from build123d import *

# Parameters (mm, degrees)
SKETCH_1_W          = 12.5
SKETCH_1_H          = 12.5
EXTRUDE_412_DEPTH   = 4.5
FILLET_1_R          = 1.5
FILLET_2_R          = 1
SKETCH_2_W          = 15
SKETCH_2_H          = 15
EXTRUDE_1329_DEPTH  = 0.5
FILLET_3_R          = 3
CUT_EXTRUDE_1_DEPTH = 0.4
FILLET_4_R          = 0.5


with BuildPart() as part:
    # Эскиз1 → Extrude 412 (new body)
    with BuildSketch(Plane.XY):
        Rectangle(SKETCH_1_W, SKETCH_1_H)
    extrude(amount=EXTRUDE_412_DEPTH)

    # Скругление1
    fillet_1_edges = [part.edges().sort_by_distance(p)[0] for p in [
        (-6.25, 6.25, 2.25),
        (6.25, 6.25, 2.25),
        (6.25, -6.25, 2.25),
        (-6.25, -6.25, 2.25),
    ]]
    fillet(fillet_1_edges, radius=FILLET_1_R)

    # Скругление2
    fillet_2_edges = [part.edges().sort_by_distance(p)[0] for p in [
        (6.25, 0, 4.5),
        (0, -6.25, 4.5),
        (-6.25, 0, 4.5),
        (0, 6.25, 4.5),
        (-5.810660172, -5.810660172, 4.5),
        (-5.810660172, 5.810660172, 4.5),
        (5.810660172, 5.810660172, 4.5),
        (5.810660172, -5.810660172, 4.5),
    ]]
    fillet(fillet_2_edges, radius=FILLET_2_R)

    # Эскиз2 → Extrude 1329 (add)
    with BuildSketch(Plane(origin=(0, 0, 0), x_dir=(-1, 0, 0), z_dir=(0, 0, -1))):
        Rectangle(SKETCH_2_W, SKETCH_2_H)
    extrude(amount=-EXTRUDE_1329_DEPTH)

    # Скругление3
    fillet_3_edges = [part.edges().sort_by_distance(p)[0] for p in [
        (7.5, -7.5, 0.25),
        (7.5, 7.5, 0.25),
        (-7.5, 7.5, 0.25),
        (-7.5, -7.5, 0.25),
    ]]
    fillet(fillet_3_edges, radius=FILLET_3_R)

    # Эскиз4 → Вырез-Вытянуть1 (cut)
    with BuildSketch(Plane.XY.offset(4.5)):
        Polygon((-3.61015121, 1.724032908), (-3.61015121, -1.724032908), (-1.580654119, -1.724032908), (0.195408328, -3.515449311), (0.195408328, 3.515449311), (-1.580654119, 1.724032908), align=None)
        with BuildLine():
            ThreePointArc((1.529185986, -1.383686517), (1.749358373, 0), (1.529185986, 1.383686517))
            ThreePointArc((1.529185986, 1.383686517), (1.758587632, 1.835514539), (2.210415654, 1.606112893))
            ThreePointArc((2.210415654, 1.606112893), (2.465980556, 0), (2.210415654, -1.606112893))
            ThreePointArc((2.210415654, -1.606112893), (1.758587632, -1.835514539), (1.529185986, -1.383686517))
        make_face()
        with BuildLine():
            ThreePointArc((2.847646844, -3.007485014), (3.609370922, 0), (2.847646844, 3.007485014))
            ThreePointArc((2.847646844, 3.007485014), (3.055453428, 3.70569516), (3.753663574, 3.497888576))
            ThreePointArc((3.753663574, 3.497888576), (4.639595154, 0), (3.753663574, -3.497888576))
            ThreePointArc((3.753663574, -3.497888576), (3.055453428, -3.70569516), (2.847646844, -3.007485014))
        make_face()
    extrude(amount=-CUT_EXTRUDE_1_DEPTH, mode=Mode.SUBTRACT)

    # Скругление4
    fillet_4_edges = [part.edges().sort_by_distance(p)[0] for p in [
        (0.195408328, 3.515449311, 4.3),
        (0.195408328, -3.515449311, 4.3),
    ]]
    fillet(fillet_4_edges, radius=FILLET_4_R)


solid = part.part
Verification items for the finished model (mm, model axes). A direction names the side the tool comes from. Give positions to 0.01 mm unless a question says otherwise; leave off trailing zeros. Write each loop counter-clockwise with the first axis right and the second up, starting at its lowest first coordinate (ties: lowest second). Pieces come first, ordered by that corner, then holes.
(1) Cross-section at B-B (y = 4.25). Enter the section's corners in (x, z), plus the area to 3 significant figures.
(2) Access from +Z, -Z, +X, -X, +Y, -Y to the whole of each face (thin tool, end or side, straight path). Record for faces 4 (the face through (0, 6.25, 2)), 5 (the face through (4, 0, 4.1)), 6 (the face through (-6.25, 0, 2)), 7 (the face through (5.82, 5.8, 2.02)), 8 (the face through (-5.82, 5.8, 2.02)).
(3) Gauge pin test, flat ends, axial feed: pin 1 (1.5 mm diameter, centred on x = -2.5, z = 2.5, fed in from +Y); pin 2 (2.5 mm diameter, centred on y = 2.5, z = 2, fed in from +X); pin 3 (0.9 mm diameter, centred on x = 2, z = 1.5, fed in from -Y). Record the tip position at first contact, or that the pin passes through.
(4) Mould release check, pull along X, two halves, no side actions. Record for faces 1 (the face through (6.64, 6.6, 0.25)), 2 (the face through (0.067, -5.949, 4.215)), 3 (the face through (2, 0, 4.1)): +X half, -X half, draft (parallel to the pull), parting line (faces both ways), or undercut.
(5) Material ranges on line 1 (X direction, y = -0.5, z = 4.25); line 2 (X direction, y = -0.5, z = 4.3); line 3 (Y direction, x = 1.25, z = 0.55), recorded low to high.
(6) Cross-section at D-D (y = 1). Enter the section's corners in (x, z), plus the area to 3 significant figures.
(7) Cross-section at A-A (z = 1.45). Enter the section's corners in (x, y), plus the area to 3 significant figures.
Worked out:
1. outline: (-7.5, 0) - (7.5, 0) - (7.5, 0.5) - (6.25, 0.5) - (6.25, 3.5) arc R1 ccw to (5.25, 4.5) - (-5.25, 4.5) arc R1 ccw to (-6.25, 3.5) - (-6.25, 0.5) - (-7.5, 0.5) - close
1. area: 57.1 mm2
2. face 4: +Z, +X, -X, +Y
2. face 5: +Z
2. face 6: +Z, -X, +Y, -Y
2. face 7: +Z, +X, +Y
2. face 8: +Z, -X, +Y
3. pin 1: stops at y = 6.25
3. pin 2: stops at x = 6.25
3. pin 3: stops at y = -6.25
4. face 1: +X half
4. face 2: draft
4. face 3: undercut
5. line 1: x = -5.91 to -3.61, 0.2 to 1.72, 2.44 to 3.59, 4.62 to 5.91
5. line 2: x = -5.85 to -3.61, 0.2 to 1.72, 2.44 to 3.59, 4.62 to 5.85
5. line 3: y = -6.25 to 6.25
6. outline: (-7.5, 0) - (7.5, 0) - (7.5, 0.5) - (6.25, 0.5) - (6.25, 3.5) arc R1 ccw to (5.25, 4.5) - (4.57, 4.5) - (4.57, 4.1) - (3.53, 4.1) - (3.53, 4.5) - (2.37, 4.5) - (2.37, 4.1) - (1.64, 4.1) - (1.64, 4.5) - (0.2, 4.5) - (0.2, 4.1) - (-3.61, 4.1) - (-3.61, 4.5) - (-5.25, 4.5) arc R1 ccw to (-6.25, 3.5) - (-6.25, 0.5) - (-7.5, 0.5) - close
6. area: 54.8 mm2
7. outline: (-6.25, -4.75) arc R1.5 ccw to (-4.75, -6.25) - (4.75, -6.25) arc R1.5 ccw to (6.25, -4.75) - (6.25, 4.75) arc R1.5 ccw to (4.75, 6.25) - (-4.75, 6.25) arc R1.5 ccw to (-6.25, 4.75) - close
7. area: 154 mm2
